```python
from build123d import *

# Parameters (mm, degrees)
BOSS_EXTRUDE1_DEPTH     = 50
BOSS_EXTRUDE2_DEPTH     = 25
CHAMFER1_SIZE           = 1
CUT_EXTRUDE1_DEPTH      = 76.208044782
CUT_EXTRUDE1_DEPTH_BACK = 76.208044782
SKETCH2_R               = 1.5
CUT_EXTRUDE2_DEPTH      = 76.208044782
CUT_EXTRUDE2_DEPTH_BACK = 4
SKETCH2_3_R             = 2.5
SKETCH2_3_R_2           = 1.5
CUT_EXTRUDE3_DEPTH      = 92.348180058
CUT_EXTRUDE3_DEPTH_BACK = 92.348180058
SKETCH3_R               = 2.5
CUT_EXTRUDE4_START      = -4.7
SKETCH3_3_R             = 5
SKETCH3_3_R_2           = 2.5
CUT_EXTRUDE4_DEPTH      = 2
FILLET1_R               = 2


with BuildPart() as part:
    # Sketch1 → Boss-Extrude1 (new, symmetric)
    with BuildSketch(Plane(origin=(0, 0, 0), x_dir=(0, 0, -1), z_dir=(1, 0, 0))):
        Polygon((25.5, 25.7), (25.5, 20), (14.5, 20), (14.5, 19), (5.5, 19), (5.5, 20), (-5.5, 20), (-5.5, 19), (-14.5, 19), (-14.5, 20), (-20.5, 20), (-20.5, 14.5), (-19.5, 14.5), (-19.5, 5.5), (-20.5, 5.5), (-20.5, 0), (-26.2, 0), (-26.2, 25.7), align=None)
    extrude(amount=BOSS_EXTRUDE1_DEPTH, both=True)

    # Sketch1<3> → Boss-Extrude2 (add, symmetric)
    with BuildSketch(Plane(origin=(0, 0, 0), x_dir=(0, 0, -1), z_dir=(1, 0, 0))):
        Polygon((32.5, 24), (25.5, 24), (25.5, 20), (52.5, 20), (52.5, 25.7), (32.5, 25.7), align=None)
    extrude(amount=BOSS_EXTRUDE2_DEPTH, both=True)

    # Chamfer1
    chamfer1_edges = [part.edges().sort_by_distance(p)[0] for p in [
        (0, 5.5, 19.5),
        (0, 14.5, 19.5),
        (0, 19, 14.5),
        (0, 19, 5.5),
        (0, 19, -5.5),
        (0, 19, -14.5),
        (-50, 10, 19.5),
        (50, 10, 19.5),
        (50, 19, 10),
        (-50, 19, 10),
        (50, 19, -10),
        (-50, 19, -10),
    ]]
    chamfer(chamfer1_edges, length=CHAMFER1_SIZE - 0.0001)  # a hair under: the kernel refuses the full size

    # Sketch2 → Cut-Extrude1 (cut, two sides: drawn at the far end of the back side and taken through both)
    with BuildSketch(Plane.XZ.offset(-20).offset(-CUT_EXTRUDE1_DEPTH_BACK)):
        with Locations(Location((-15, -42, 0), (0, 0, 270))):
            Circle(SKETCH2_R)
        with Locations(Location((15, -42, 0), (0, 0, 270))):
            Circle(SKETCH2_R)
        with Locations(Location((-15, -12, 0), (0, 0, 270))):
            Circle(SKETCH2_R)
        with Locations(Location((15, -12, 0), (0, 0, 270))):
            Circle(SKETCH2_R)
    extrude(amount=CUT_EXTRUDE1_DEPTH + CUT_EXTRUDE1_DEPTH_BACK, mode=Mode.SUBTRACT)

    # Sketch2<3> → Cut-Extrude2 (cut, two sides: drawn at the far end of the back side and taken through both)
    # profile 1 of 4: a face of its own
    with BuildSketch(Plane.XZ.offset(-20).offset(-CUT_EXTRUDE2_DEPTH_BACK)):
        with Locations(Location((-15, -12, 0), (0, 0, 270))):
            Circle(SKETCH2_3_R)
        with Locations(Location((-15, -12, 0), (0, 0, 270))):
            Circle(SKETCH2_3_R_2, mode=Mode.SUBTRACT)
    # profile 2 of 4: a face of its own
    with BuildSketch(Plane.XZ.offset(-20).offset(-CUT_EXTRUDE2_DEPTH_BACK)):
        with Locations(Location((-15, -42, 0), (0, 0, 90))):
            Circle(SKETCH2_3_R)
        with Locations(Location((-15, -42, 0), (0, 0, 270))):
            Circle(SKETCH2_3_R_2, mode=Mode.SUBTRACT)
    # profile 3 of 4: a face of its own
    with BuildSketch(Plane.XZ.offset(-20).offset(-CUT_EXTRUDE2_DEPTH_BACK)):
        with Locations(Location((15, -42, 0), (0, 0, 90))):
            Circle(SKETCH2_3_R)
        with Locations(Location((15, -42, 0), (0, 0, 270))):
            Circle(SKETCH2_3_R_2, mode=Mode.SUBTRACT)
    # profile 4 of 4: a face of its own
    with BuildSketch(Plane.XZ.offset(-20).offset(-CUT_EXTRUDE2_DEPTH_BACK)):
        with Locations(Location((15, -12, 0), (0, 0, 90))):
            Circle(SKETCH2_3_R)
        with Locations(Location((15, -12, 0), (0, 0, 270))):
            Circle(SKETCH2_3_R_2, mode=Mode.SUBTRACT)
    extrude(amount=CUT_EXTRUDE2_DEPTH + CUT_EXTRUDE2_DEPTH_BACK, mode=Mode.SUBTRACT)

    # Sketch3 → Cut-Extrude3 (cut, two sides: drawn at the far end of the back side and taken through both)
    with BuildSketch(Plane(origin=(0, 0, 19.5), x_dir=(-1, 0, 0), z_dir=(0, 0, -1)).offset(-CUT_EXTRUDE3_DEPTH_BACK)):
        with Locations((-40, 10)):
            Circle(SKETCH3_R)
        with Locations((40, 10)):
            Circle(SKETCH3_R)
    extrude(amount=CUT_EXTRUDE3_DEPTH + CUT_EXTRUDE3_DEPTH_BACK, mode=Mode.SUBTRACT)

    # Sketch3<3> → Cut-Extrude4 (cut)
    # profile 1 of 2: a face of its own
    with BuildSketch(Plane(origin=(0, 0, 19.5), x_dir=(-1, 0, 0), z_dir=(0, 0, -1)).offset(CUT_EXTRUDE4_START)):
        with Locations(Location((-40, 10, 0), (0, 0, 180))):
            Circle(SKETCH3_3_R)
        with Locations((-40, 10)):
            Circle(SKETCH3_3_R_2, mode=Mode.SUBTRACT)
    # profile 2 of 2: a face of its own
    with BuildSketch(Plane(origin=(0, 0, 19.5), x_dir=(-1, 0, 0), z_dir=(0, 0, -1)).offset(CUT_EXTRUDE4_START)):
        with Locations(Location((40, 10, 0), (0, 0, 180))):
            Circle(SKETCH3_3_R)
        with Locations((40, 10)):
            Circle(SKETCH3_3_R_2, mode=Mode.SUBTRACT)
    extrude(amount=-CUT_EXTRUDE4_DEPTH, mode=Mode.SUBTRACT)

    # Fillet1
    fillet1_edges = [part.edges().sort_by_distance(p)[0] for p in [
        (50, 12.85, 26.2),
        (-50, 12.85, 26.2),
        (-50, 22.85, -25.5),
        (50, 22.85, -25.5),
        (25, 22.85, -52.5),
        (-25, 22.85, -52.5),
    ]]
    fillet(fillet1_edges, radius=FILLET1_R)


solid = part.part
```
Work out the finished part from the listing and answer in its coordinate system (mm). A direction names the side the tool comes from. Round coordinates to 2 decimals unless told otherwise and drop trailing zeros. Loops run counter-clockwise (first coordinate to the right, second up) from the corner with the lowest first, then second, coordinate; pieces in that order, holes last. Notation, with made-up numbers: M 55.5,29.25 L 108.5,29.25 A27 cw 108.5,57.25 Z; hole C -19,-4 d3. An arc over 180 degrees is marked long. One line per question, with ' | ' between items.
Q1. Consider line 1 along X through (y, z) = (24.4, -42); line 2 along Z through (x, y) = (-15, 20.75); line 3 along X through (y, z) = (10, 22.5). Determine where each line is inside the solid, lowest interval first. Write a range as from..to.
Conclusion:
line 1: x = -25..-16.5, -13.5..13.5, 16.5..25 | line 2: z = -52.5..-44.5, -39.5..-14.5, -9.5..26.2 | line 3: x = -50..-42.5, -37.5..37.5, 42.5..50
Q2. Find section C-C, the plane y = 10. Give the vertices of the cut face in (x, z), then the cut area to 3 significant figures.
Conclusion:
outline: M -50,20.5 L -49,19.5 L -42.5,19.5 L -42.5,24.2 L -45,24.2 L -45,26.2 L -48,26.2 A2 ccw -50,24.2 Z; M -37.5,19.5 L 37.5,19.5 L 37.5,24.2 L 35,24.2 L 35,26.2 L -35,26.2 L -35,24.2 L -37.5,24.2 Z; M 42.5,19.5 L 49,19.5 L 50,20.5 L 50,24.2 A2 ccw 48,26.2 L 45,26.2 L 45,24.2 L 42.5,24.2 Z | area: 580 mm2
Q3. The mould has two halves that part along X. Classify faces 1 (the flat face through (50, 21, 4)), 2 (the flat face through (1, 19, -10)), 3 (the flat face through (17, 24, -42)): +X half, -X half, draft (parallel to the pull), parting line (faces both ways), or undercut.
Conclusion:
face 1: +X half | face 2: draft | face 3: undercut
Q4. Find section D-D, the plane y = 2.75. Give the vertices of the cut face in (x, z), then the cut area to 3 significant figures.
Conclusion:
outline: M -50,20.5 L 50,20.5 L 50,24.2 A2 ccw 48,26.2 L -48,26.2 A2 ccw -50,24.2 Z | area: 568 mm2
Q5. Each of these flat-tipped pins is pushed along its axis until it touches: pin 1 Ø2.5 at (x, z) = (15, -12) entering from -Y; pin 2 Ø3 at (x, y) = (-31, 14.5) entering from -Z; pin 3 Ø4 at (x, z) = (-15, -13) entering from -Y; pin 4 Ø7.5 at (x, z) = (15, 10) entering from -Y. Where does it stop, or does it pass through?
Conclusion:
pin 1: passes through | pin 2: stops at z = 19.5 | pin 3: stops at y = 19.12 | pin 4: stops at y = 19
Q6. Find section B-B, the plane z = -42. Give the vertices of the cut face in (x, y).
Conclusion:
outline: M -25,20 L -17.5,20 L -17.5,24 L -16.5,24 L -16.5,25.7 L -25,25.7 Z; M -13.5,24 L -12.5,24 L -12.5,20 L 12.5,20 L 12.5,24 L 13.5,24 L 13.5,25.7 L -13.5,25.7 Z; M 16.5,24 L 17.5,24 L 17.5,20 L 25,20 L 25,25.7 L 16.5,25.7 Z
Q7. A tool of negligible diameter and unlimited length cuts with its end or side. For faces 4 (the cylindrical face through (-14.04, 22.03, -39.69)), 5 (the flat face through (0.7, 24.2, -25.5)), 6 (the cylindrical face through (35, 10, 25)), from which of +Z, -Z, +X, -X, +Y, -Y can it reach the whole face along a straight path? Write none if from no direction.
Conclusion:
face 4: -Y | face 5: +Y | face 6: +Z
